For this review, take the finished solid that the model builds, in its own axes (mm). Face numbers are marked on the shaded views. A direction names the side the tool comes from. Coordinates: 2 decimals unless noted, no trailing zeros. Order: outer loops, then holes, each group sorted by start corner. A loop starts at its lowest first (then second) coordinate and runs counter-clockwise, first axis right, second up. Notation, with made-up numbers: (56, -34.75) -> (68, -34.75) arc R9 cw to (68, -29.75) -> close; hole circle Ø7 at (72.5, -37.75). An arc over 180 degrees is marked (long way). Write item = value, one per line. Start each with the question number.
1) Consider section B-B on z = -10. Give the boundary of the cut face in (x, y).
2) Machinability: for the marked faces 1, 2 and 3, which of the approach directions +Z, -Z, +X, -X, +Y, -Y give a long, thin tool a straight path to every point of the face, cutting with its end or side? Answer none if there is none.
3) Wall thickness on probe 1 along X at (y, z) = (-24.5, 26.5); probe 2 along Y at (x, z) = (61, -70); probe 3 along Z at (x, y) = (-29.5, 25.5): over which ranges is each line inside the solid? List them lowest first. Write a range as [from, to].
4) Consider section A-A on y = 38.5. Give the boundary of the cut face in (x, z).
5) Consider section C-C on x = 45.5. Give the boundary of the cut face in (y, z).
6) Consider section D-D on z = 62. Give the boundary of the cut face in (x, y), and give its area (3 significant figures).
7) Insertion check: pin 1 Ø23 at (y, z) = (35, 46) entering from +X; pin 2 Ø4 at (x, y) = (-30.5, 8.5) entering from +Z. Each pin has a flat end and moves straight along its axis. Give the tip position at first contact, or say it passes through.
from build123d import *

# Parameters (mm, degrees)
F0_W     = 228.6
F0_H     = 152.4
F1_DEPTH = 76.2
F2_W     = 165.1
F2_H     = 76.2
F3_DEPTH = 152.401
F4_W     = 101.6
F4_H     = 76.2
F5_DEPTH = 50.8


with BuildPart() as f1:
    # F0 (on Front) → F1 (new body, symmetric)
    with BuildSketch(Plane.XZ):
        Rectangle(F0_W, F0_H)
    extrude(amount=F1_DEPTH, both=True)

    # F2 (on face) → F3 (cut, through all)
    with BuildSketch(Plane.XZ.offset(76.2)):
        with Locations((31.75, 38.1)):
            Rectangle(F2_W, F2_H)
    extrude(amount=-F3_DEPTH, mode=Mode.SUBTRACT)

    # F4 (on face) → F5 (cut)
    with BuildSketch(Plane.XZ.offset(76.2)):
        with Locations((63.5, -38.1)):
            Rectangle(F4_W, F4_H)
    extrude(amount=-F5_DEPTH, mode=Mode.SUBTRACT)


solid = f1.part
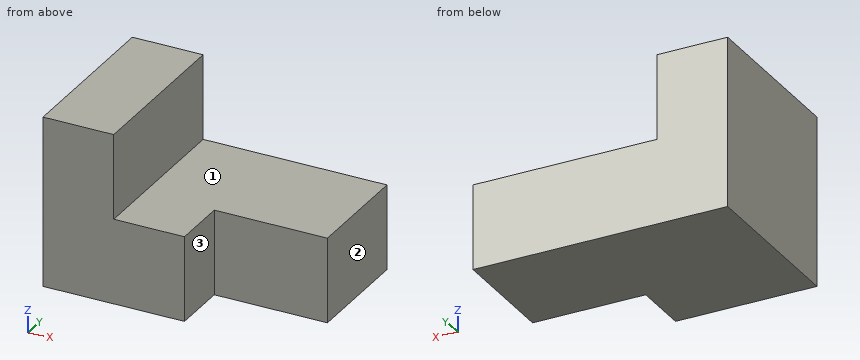
Answer sheet:
q1.outline = (-114.3, -76.2) -> (12.7, -76.2) -> (12.7, -25.4) -> (114.3, -25.4) -> (114.3, 76.2) -> (-114.3, 76.2) -> close
q2.face_1 = +Z, +X, +Y, -Y
q2.face_2 = +Z, -Z, +X, +Y, -Y
q2.face_3 = +Z, -Z, +X, -Y
q3.probe_1 = [-114.3, -50.8]
q3.probe_2 = [-25.4, 76.2]
q3.probe_3 = [-76.2, 0]
q4.outline = (-114.3, -76.2) -> (114.3, -76.2) -> (114.3, 0) -> (-50.8, 0) -> (-50.8, 76.2) -> (-114.3, 76.2) -> close
q5.outline = (-25.4, -76.2) -> (76.2, -76.2) -> (76.2, 0) -> (-25.4, 0) -> close
q6.outline = (-114.3, -76.2) -> (-50.8, -76.2) -> (-50.8, 76.2) -> (-114.3, 76.2) -> close
q6.area = 9,680 mm2
q7.pin_1 = -50.8
q7.pin_2 = 0
